The listing builds one solid part. Answer for the finished solid, in the listing's coordinates (mm). Face numbers are marked on the shaded views. Coordinates: 2 decimals unless noted, no trailing zeros. Order: outer loops, then holes, each group sorted by start corner. A loop starts at its lowest first (then second) coordinate and runs counter-clockwise, first axis right, second up.
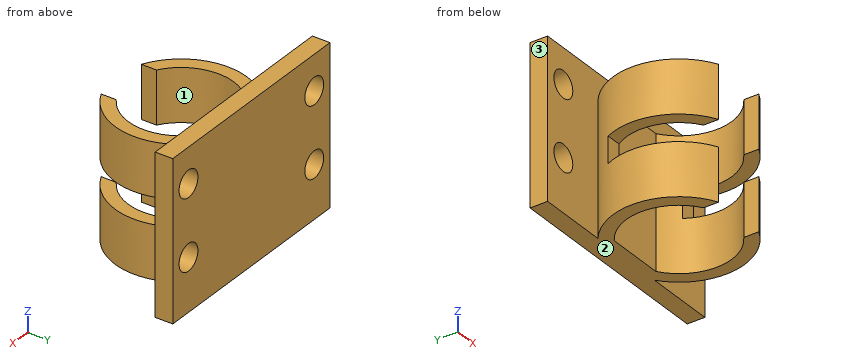
from build123d import *

# Parameters (mm, degrees)
EXTRUDE_1_DEPTH     = 15
CUT_EXTRUDE_1_DEPTH = 7.5
EXTRUDE_3_DEPTH     = 18
SKETCH_3_R          = 1.5
CUT_EXTRUDE_2_DEPTH = 10


with BuildPart() as part:
    # Sketch 1 → Extrude 1 (new body)
    with BuildSketch(Plane.XY):
        with BuildLine():
            ThreePointArc((3.195328917, -6.785268831), (7.461194526, -0.761955539), (4.500921435, 5.999308813))
            Line((4.500921435, 5.999308813), (-4.500433628, 5.999674755))
            ThreePointArc((-4.500433628, 5.999674755), (-7.461256455, -0.761348873), (-3.195880618, -6.785008996))
            Line((-3.195880618, -6.785008996), (-3.195880618, -5.078025903))
            ThreePointArc((-3.195880618, -5.078025903), (-5.999570878, -0.071758494), (-3.316421512, 5.000134834))
            Line((-3.316421512, 5.000134834), (3.316828063, 4.999865158))
            ThreePointArc((3.316828063, 4.999865158), (5.999565023, -0.07224632), (3.195467712, -5.078285744))
            Line((3.195467712, -5.078285744), (3.195328917, -6.785268831))
        make_face()
    extrude(amount=EXTRUDE_1_DEPTH)

    # Sketch 2 → Cut-Extrude 1 (cut, symmetric)
    with BuildSketch(Plane(origin=(0, 0, 0), x_dir=(0, 0, -1), z_dir=(1, 0, 0))):
        Polygon((-7.5, -6.785268831), (-6, -6.785268831), (-6, 3.214731169), (-9, 3.214731169), (-9, -6.785268831), align=None)
    extrude(amount=CUT_EXTRUDE_1_DEPTH, both=True, mode=Mode.SUBTRACT)

    # Sketch 1_4 → Extrude 3 (add)
    with BuildSketch(Plane.XY):
        Polygon((12.500650474, 7.999329111), (-12.500650425, 8.000345629), (-12.500650425, 5.999999996), (12.500487826, 5.998983598), align=None)
    extrude(amount=EXTRUDE_3_DEPTH)

    # Sketch 3 → Cut-Extrude 2 (cut)
    with BuildSketch(Plane(origin=(0.000325262, 7.999837357, 0), x_dir=(0.999999999, -4.0659e-05, 0), z_dir=(4.0659e-05, 0.999999999, 0))):
        with Locations((-10.000975697, -6)):
            Circle(SKETCH_3_R)
        with Locations((-10.000975697, -14)):
            Circle(SKETCH_3_R)
        with Locations((10.000867281, -6.000271056)):
            Circle(SKETCH_3_R)
        with Locations((10.000650456, -14.000271053)):
            Circle(SKETCH_3_R)
    extrude(amount=-CUT_EXTRUDE_2_DEPTH, mode=Mode.SUBTRACT)


solid = part.part
(1) Find section D-D on y = 4.5. Determine the outline of the cut face in (x, z).
(2) Find the intervals of material crossed by probe 1 along X at (y, z) = (6.45, 14); probe 2 along X at (y, z) = (0, 3); probe 3 along Z at (x, y) = (5, -5), in increasing order.
(3) Find section A-A on x = -6.5. Determine the outline of the cut face in (y, z).
(4) Find section B-B on y = -1. Determine the outline of the cut face in (x, z).
(5) The mould has two halves that part along X. Classify the marked faces 1, 2 and 3: pulls with the +X half, pulls with the -X half, needs draft (parallel to the pull), parting line crosses it, or undercut.
(6) Given pin 1 Ø0.5 at (y, z) = (-6, 10.5) entering from -X; pin 2 Ø4 at (y, z) = (-4.5, 16) entering from +X; pin 3 Ø0.5 at (x, z) = (6, 7.5) entering from -Y, each flat-ended and moving along its own axis, determine where each tip first touches the part or whether it passes through.
(7) Find section C-C on x = 4. Determine the outline of the cut face in (y, z), then the cut area to 3 significant figures.
Resolved:
1. outline: (-6, 0) - (-3.97, 0) - (-3.97, 15) - (-6, 15) - close; (3.97, 0) - (6, 0) - (6, 15) - (3.97, 15) - close
2. probe 1: x = -12.5 to -11.5, -8.5 to 8.5, 11.5 to 12.5
2. probe 2: x = -7.5 to -6, 6 to 7.5
2. probe 3: z = 0 to 6, 9 to 15
3. outline: (-3.74, 0) - (3.74, 0) - (3.74, 15) - (-3.74, 15) - (-3.74, 9) - (3.21, 9) - (3.21, 6) - (-3.74, 6) - close; (6, 0) - (8, 0) - (8, 18) - (6, 18) - close
4. outline: (-7.43, 0) - (-5.92, 0) - (-5.92, 6) - (-7.43, 6) - close; (-7.43, 9) - (-5.92, 9) - (-5.92, 15) - (-7.43, 15) - close; (5.92, 0) - (7.43, 0) - (7.43, 6) - (5.92, 6) - close; (5.92, 9) - (7.43, 9) - (7.43, 15) - (5.92, 15) - close
5. face 1: undercut
5. face 2: needs draft
5. face 3: pulls with the -X half
6. pin 1: stops at x = -4.82
6. pin 2: stops at x = 6.97
6. pin 3: stops at y = 3.21
7. outline: (-6.34, 0) - (-4.47, 0) - (-4.47, 6) - (-6.34, 6) - close; (-6.34, 9) - (-4.47, 9) - (-4.47, 15) - (-6.34, 15) - close; (4.47, 0) - (8, 0) - (8, 18) - (6, 18) - (6, 15) - (4.47, 15) - close
7. area: 81.4 mm2
